Build history of the part. All positions in model axes, mm. A direction names the side the tool comes from. Round coordinates to 2 decimals unless told otherwise and drop trailing zeros. Write each loop counter-clockwise with the first axis right and the second up, starting at its lowest first coordinate (ties: lowest second). Pieces come first, ordered by that corner, then holes. Notation, with made-up numbers: (-30.5, 59) - (-23.5, 59) arc R19 ccw to (-23.5, 86) - close; hole circle Ø9 at (-17, -36.75). An arc over 180 degrees is marked (long way). Answer as a JSON object with one key per item and string values. Group by question number.
Item 1: Flat gauge pins, fed straight in: pin 1 (6 mm diameter, centred on x = 3, z = 3.5, fed in from -Y); pin 2 (0.8 mm diameter, centred on x = 0.5, y = 1.5, fed in from -Z); pin 3 (3 mm diameter, centred on x = -0.5, z = 0.5, fed in from +Y). Where does each tip first touch, or does it go through?
Item 2: Slice it at B-B, the plane z = 3.5. List the corners of the cut face in (x, y).
Item 3: Two-plate mould, pull along Y, no slides. Class faces 5 (the flat face through (0, 4, 1)), 6 (the cylindrical face through (-7.215, 5.479, 5.051)), 7 (the cylindrical face through (0.17, 3.29, -1.57)): +Y half, -Y half, draft (parallel to the pull), parting line (faces both ways), or undercut.
Item 4: Probe line 1 (Z direction, x = -2.25, y = 6.25); line 2 (Y direction, x = 0, z = -2); line 3 (Y direction, x = 0, z = -3.75). List the from-to ranges inside material, lowest first. Write a range as from..to.
Item 5: Slice it at D-D, the plane y = 2. List the corners of the cut face in (x, z), then the cut area to 3 significant figures.
Item 6: Slice it at C-C, the plane x = 6. List the corners of the cut face in (y, z).
Item 7: Which spindle directions (+Z, -Z, +X, -X, +Y, -Y) get a long thin tool onto all of the face, cutting with end or side? Do faces 1 (the cylindrical face through (7.199, 5.479, 5.035)), 2 (the cylindrical face through (7.199, 3.549, -6.465)), 3 (the flat face through (0, 6, 4.75)), 4 (the cylindrical face through (-7.215, 5.479, -3.051)). Say none if no direction does.
from build123d import *

# Parameters (mm, degrees)
SKETCH1_W           = 15
SKETCH1_H           = 13.5
BOSS_EXTRUDE1_DEPTH = 7
SKETCH2_W           = 15
SKETCH2_H           = 7.5
CUT_EXTRUDE2_DEPTH  = 3
SKETCH3_R           = 1.3
CUT_EXTRUDE3_DEPTH  = 10.5
FILLET1_R           = 1


with BuildPart() as part:
    # Sketch1 → Boss-Extrude1 (new body)
    with BuildSketch(Plane(origin=(0, 0, 0), x_dir=(1, 0, 0), z_dir=(0, 1, 0))):
        Rectangle(SKETCH1_W, SKETCH1_H)
    extrude(amount=BOSS_EXTRUDE1_DEPTH)

    # Sketch2 → Cut-Extrude2 (cut)
    with BuildSketch(Plane(origin=(0, 7, 0), x_dir=(1, 0, 0), z_dir=(0, 1, 0))):
        with Locations((0, -1)):
            Rectangle(SKETCH2_W, SKETCH2_H)
    extrude(amount=-CUT_EXTRUDE2_DEPTH, mode=Mode.SUBTRACT)

    # Sketch3 → Cut-Extrude3 (cut)
    with BuildSketch(Plane(origin=(0, 0, -6.75), x_dir=(-1, 0, 0), z_dir=(0, 0, -1))):
        with Locations((0, 2)):
            Circle(SKETCH3_R)
    extrude(amount=-CUT_EXTRUDE3_DEPTH, mode=Mode.SUBTRACT)

    # Fillet1
    fillet1_edges = [part.edges().sort_by_distance(p)[0] for p in [
        (7.5, 5.5, -2.75),
        (7.5, 5.5, 4.75),
        (-7.5, 5.5, 4.75),
        (-7.5, 5.5, -2.75),
        (7.5, 3.5, 6.75),
        (-7.5, 3.5, 6.75),
        (-7.5, 3.5, -6.75),
        (7.5, 3.5, -6.75),
    ]]
    fillet(fillet1_edges, radius=FILLET1_R - 0.0001)  # a hair under: the kernel refuses the full size


solid = part.part
Geometry says:
{
 "1": {"pin 1": "stops at y = 0", "pin 2": "stops at z = 3.75", "pin 3": "stops at y = 4"},
 "2": {"outline": "(-7.5, 0) - (7.5, 0) - (7.5, 4) - (-7.5, 4) - close; hole circle Ø2.6 at (0, 2)"},
 "3": {"face 5": "+Y half", "face 6": "draft", "face 7": "undercut"},
 "4": {"line 1": "z = -6.75..-2.75, 4.75..6.75", "line 2": "y = 0..0.7, 3.3..4", "line 3": "y = 0..0.7, 3.3..7"},
 "5": {"outline": "(-7.5, -5.75) arc R1 ccw to (-6.5, -6.75) - (-1.3, -6.75) - (-1.3, 3.75) - (1.3, 3.75) - (1.3, -6.75) - (6.5, -6.75) arc R1 ccw to (7.5, -5.75) - (7.5, 5.75) arc R1 ccw to (6.5, 6.75) - (-6.5, 6.75) arc R1 ccw to (-7.5, 5.75) - close", "area": "174 mm^2"},
 "6": {"outline": "(0, -6.75) - (7, -6.75) - (7, -2.75) - (4, -2.75) - (4, 4.75) - (7, 4.75) - (7, 6.75) - (0, 6.75) - close"},
 "7": {"face 1": "+X, +Y", "face 2": "-Z, +X, +Y, -Y", "face 3": "+X, -X, +Y", "face 4": "-X, +Y"}
}
